Could you check a few things on this model? Use its own coordinates, in mm. A direction names the side the tool comes from. Round coordinates to 2 decimals unless told otherwise and drop trailing zeros. Write each loop counter-clockwise with the first axis right and the second up, starting at its lowest first coordinate (ties: lowest second). Pieces come first, ordered by that corner, then holes. Notation, with made-up numbers: (38.5, 50.5) - (71.5, 50.5) arc R27 ccw to (71.5, 82.5) - close; hole circle Ø4 at (-35, 47.5). An arc over 180 degrees is marked (long way). Write each question's results on one line, items separated by ' | '. Start each with the question number.
(1) On a 3-axis mill with a long thin cutter (end or side, diameter ignored), from which of +Z, -Z, +X, -X, +Y, -Y can I reach the whole of each face in a straight line? I mean faces 4 (the flat face through (3.131, 17.104, 25.137)), 5 (the flat face through (3, -3, 50.8)), 6 (the flat face through (3, -3, -50.8)). Say none if no direction works.
(2) Imagine slicing it at C-C on x = 4.5. State how many separate pieces and enclosed holes the cut face has, then the cut area to 3 significant figures.
(3) For P1, Ø0.8, axis at x = 3, z = -43.5, coming from the +Y side; P2, Ø5, axis at y = 20.5, z = -12.5, coming from the -X side; P3, Ø3, axis at x = 2.5, z = 28.5, coming from the -Y side; P4, Ø1.5, axis at x = 5, y = 24.5, coming from the +Z side, each with a flat end and sliding along its axis, tell me the tip position at first contact or that it passes through.
(4) Imagine slicing it at A-A on z = 0. Write out the boundary of the cut face in (x, y).
(5) Imagine slicing it at B-B on y = 15. Write out the boundary of the cut face in (x, z).
(6) Thinking about a two-plate mould opening in Y: for faces 1 (the cylindrical face through (3.13, 12.36, 51.84)), 2 (the flat face through (3, -6.35, -47)), 3 (the cylindrical face through (3.131, 8.533, 43.954)), which applies, +Y half, -Y half, draft (parallel to the pull), parting line (faces both ways), or undercut?
(7) Imagine slicing it at D-D on z = 11. Write out the boundary of the cut face in (x, y), then the cut area to 3 significant figures.
(8) Please list where these lines run through material, in increasing order: line 1 (Z direction, x = 5.5, y = 5); line 2 (Y direction, x = 2, z = 0); line 3 (Z direction, x = 4.25, y = -3.5). Write a range as [from, to].
```python
from build123d import *

# Parameters (mm, degrees)
BOSS_EXTRUDE1_DEPTH = 6.35
SKETCH2_R           = 0.1984375
CUT_EXTRUDE1_DEPTH  = 63.980878762
FILLET5_R           = 3.175
FILLET6_R           = 12.7
FILLET7_R           = 6.35
SKETCH5_R           = 2.38125
CUT_EXTRUDE6_DEPTH  = 63.697383663


with BuildPart() as part:
    # Sketch1 → Boss-Extrude1 (new body)
    with BuildSketch(Plane(origin=(0, 0, 0), x_dir=(0, 0, -1), z_dir=(1, 0, 0))):
        Polygon((50.8, -6.35), (50.8, 0), (52.3875, 0), (52.3875, 12.7), (6.35, 31.75), (0, 34.377586207), (-6.35, 31.75), (-52.3875, 12.7), (-52.3875, 0), (-50.8, 0), (-50.8, -6.35), (-44.25, -6.35), (-44.25, 0), (-42.6625, 0), (-42.6625, 6.35), (-44.25, 6.35), (-46.0375, 8.455417024), (-5.088091142, 25.4), (5.088091142, 25.4), (46.0375, 8.455417024), (44.25, 6.35), (42.6625, 6.35), (42.6625, 0), (44.25, 0), (44.25, -6.35), align=None)
    extrude(amount=BOSS_EXTRUDE1_DEPTH)

    # Sketch2 → Cut-Extrude1 (cut, through all)
    with BuildSketch(Plane(origin=(6.35, 0, 0), x_dir=(0, 0, -1), z_dir=(1, 0, 0))):
        with Locations((-50.8, 0)):
            Circle(SKETCH2_R)
        with Locations((-44.25, 0)):
            Circle(SKETCH2_R)
        with Locations(Location((44.45, 0, 0), (0, 0, 180))):
            Circle(SKETCH2_R)
        with Locations((50.8, 0)):
            Circle(SKETCH2_R)
    extrude(amount=-CUT_EXTRUDE1_DEPTH, mode=Mode.SUBTRACT)

    # Fillet5
    # the kernel refuses this fillet: 3.175 mm, written as the material it adds along each edge
    with BuildSketch(Plane(origin=(0, 8.455417024, 46.0375), x_dir=(0, 0.38235179272629993, -0.9240168324218908), z_dir=(1, 0, 0))) as fillet5_piece_1:
        with BuildLine():
            CenterArc((3.974351986, -3.175), FILLET5_R, 90, 80.095777378)
            Line((0.846670114, -2.628894599), (0, 0))
            Line((0, 0), (3.974351986, 0))
        make_face()
    extrude(amount=6.35)
    with BuildSketch(Plane(origin=(0, 8.455417024, -46.0375), x_dir=(0, -0.7623151990147004, 0.6472059466284111), z_dir=(1, 0, 0))) as fillet5_piece_2:
        with BuildLine():
            CenterArc((4.240495318, -2.80967937), FILLET5_R, 117.756060194, 80.095777378)
            Line((1.218363855, -3.782996593), (0, 0))
            Line((0, 0), (2.761872027, 0))
        make_face()
    extrude(amount=6.35)
    # the kernel refuses this fillet: 3.175 mm, written as the material it takes off along each edge
    with BuildSketch(Plane(origin=(-5.30572872, 12.7, -52.3875), x_dir=(0, -1, 0), z_dir=(1, 0, 0)), Plane(origin=(-5.30572872, 12.7, 52.3875), x_dir=(0, 0.38235179272628034, -0.9240168324218988), z_dir=(1, 0, 0))) as fillet5_2_piece_1:
        with BuildLine():
            CenterArc((FILLET5_R * 0.668438263895, -FILLET5_R), FILLET5_R, 90, 67.520565603)
            Line((-FILLET5_R * 0.255578568527, -FILLET5_R * 0.617648207274), (0, 0))
            Line((0, 0), (FILLET5_R * 0.668438263895, 0))
        make_face()
    extrude(amount=16.961457439, mode=Mode.SUBTRACT)

    # Fillet6
    fillet6_edges = [part.edges().sort_by_distance(p)[0] for p in [
        (3.175, 25.4, -5.088091142),
        (3.175, 25.4, 5.088091142),
    ]]
    fillet(fillet6_edges, radius=FILLET6_R)

    # Fillet7
    fillet7_edges = [part.edges().sort_by_distance(p)[0] for p in [
        (3.175, 34.377586207, 0),
    ]]
    fillet(fillet7_edges, radius=FILLET7_R)

    # Sketch5 → Cut-Extrude6 (cut, through all)
    with BuildSketch(Plane(origin=(6.35, 0, 0), x_dir=(0, 0, -1), z_dir=(1, 0, 0))):
        with Locations((0, 29.092917024)):
            Circle(SKETCH5_R)
    extrude(amount=-CUT_EXTRUDE6_DEPTH, mode=Mode.SUBTRACT)


solid = part.part
```
Response:
1) face 4: +X, -X, -Y | face 5: +Z, +X, -X, -Y | face 6: -Z, +X, -X, -Y
2) separate pieces: 1 | enclosed holes: 2 | area: 938 mm²
3) P1: y = 16.54 | P2: x = 0 | P3: y = 15.09 | P4: z = 25.68
4) outline: (0, 25.4) - (6.35, 25.4) - (6.35, 26.71) - (0, 26.71) - close; (0, 31.47) - (6.35, 31.47) - (6.35, 33.86) - (0, 33.86) - close
5) outline: (0, -46.83) - (6.35, -46.83) - (6.35, -30.22) - (0, -30.22) - close; (0, 30.22) - (6.35, 30.22) - (6.35, 46.83) - (0, 46.83) - close
6) face 1: +Y half | face 2: -Y half | face 3: undercut
7) outline: (0, 22.95) - (6.35, 22.95) - (6.35, 29.83) - (0, 29.83) - close | area: 43.6 mm²
8) line 1: [-52.39, -42.66], [42.66, 52.39] | line 2: [25.4, 26.71], [31.47, 33.86] | line 3: [-50.8, -44.25], [44.25, 50.8]
